from build123d import *

# Parameters (mm, degrees)
F1_DEPTH = 2
F2_R     = 2
F3_R     = 3.175
F4_DEPTH = 2
F5_W     = 50
F5_H     = 15
F6_DEPTH = 2


with BuildPart() as f1:
    # F0 (on Top) → F1 (new body)
    with BuildSketch(Plane.XY):
        Polygon((-8, -15), (8, -15), (8, 0), (25, 0), (25, 15), (-25, 15), (-25, 0), (-8, 0), align=None)
    extrude(amount=F1_DEPTH)

    # F2
    f2_edges = [f1.edges().sort_by_distance(p)[0] for p in [
        (-8, 0, 1),
        (8, 0, 1),
    ]]
    fillet(f2_edges, radius=F2_R)

    # F3 (on face) → F4 (join)
    with BuildSketch(Plane.XY.offset(2)):
        with BuildLine():
            ThreePointArc((-13.825, 7.5), (-17, 10.675), (-20.175, 7.5))
            ThreePointArc((-20.175, 7.5), (-17, 4.325), (-13.825, 7.5))
        make_face()
        with Locations((17, 7.5)):
            Circle(F3_R)
    extrude(amount=F4_DEPTH)

    # F5 (on face) → F6 (join)
    with BuildSketch(Plane(origin=(0, 0, 0), x_dir=(1, 0, 0), z_dir=(0, 0, -1))):
        with BuildLine():
            Line((8, 2), (8, 15))
            Line((8, 15), (-8, 15))
            Line((-8, 15), (-8, 2))
            ThreePointArc((-8, 2), (-8.585786, 0.585786), (-10, 0))
            Line((-10, 0), (-25, 0))
            Line((-25, 0), (-25, -15))
            Line((-25, -15), (25, -15))
            Line((25, -15), (25, 0))
            Line((25, 0), (10, 0))
            ThreePointArc((10, 0), (8.585786, 0.585786), (8, 2))
        make_face()
        with Locations((0, -22.5)):
            Rectangle(F5_W, F5_H)
    extrude(amount=F6_DEPTH)


solid = f1.part
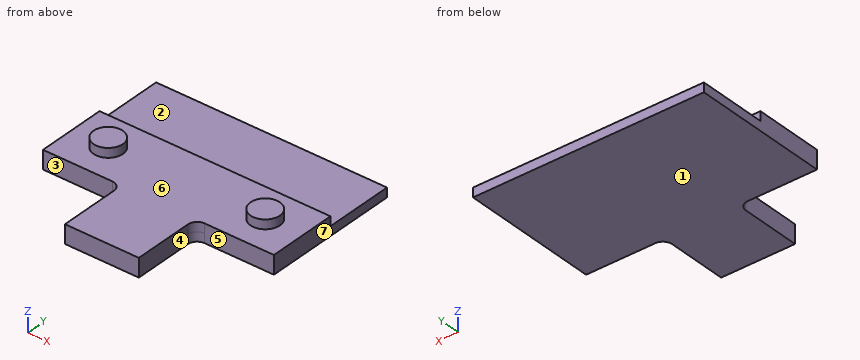
Could you check a few things on this model? Use its own coordinates, in mm. Face numbers are marked on the shaded views. A direction names the side the tool comes from. Give positions to 0.01 mm unless a question says otherwise; leave off trailing zeros. Write each loop counter-clockwise with the first axis right and the second up, starting at its lowest first coordinate (ties: lowest second). Pieces come first, ordered by that corner, then holes. Notation, with made-up numbers: (71.5, -12) -> (110.5, -12) arc R21 ccw to (110.5, 24) -> close; hole circle Ø2 at (-21.75, 77). An arc over 180 degrees is marked (long way). Write each question's results on one line, items separated by ' | '. Start each with the question number.
Q1. We'd pull the mould along X, two halves only. Please class the marked faces 5, 6 and 7: +X half, -X half, draft (parallel to the pull), parting line (faces both ways), or undercut.
Q2. Suppose I cut it at B-B, the plane z = 1.2. List the corners of the cut face in (x, y) for me, and give its area (3 significant figures).
Q3. Suppose I cut it at D-D, the plane x = 4. List the corners of the cut face in (y, z) for me.
Q4. I need wall thicknesses on probe 1 along Y at (x, z) = (-13.5, -0.15); probe 2 along Z at (x, y) = (11, 14); probe 3 along Z at (x, y) = (4, 20.5). Which ranges of each line are inside material? Lowest first, please.
Q5. I'm going to push flat-ended pins straight in: pin 1 Ø3 at (x, z) = (20.5, 0.5) entering from -Y; pin 2 Ø4.5 at (x, y) = (-4, 25.5) entering from +Z; pin 3 Ø2 at (y, z) = (-10, -0.5) entering from +X; pin 4 Ø24 at (x, y) = (-5, 3.5) entering from +Z. Where does each tip first touch, or does it pass through?
Q6. Which directions (+Z, -Z, +X, -X, +Y, -Y) give clear straight access to the entire face, cutting with the end or side of a thin tool? Please do the marked faces 1, 2, 3 and 4.
Q7. Suppose I cut it at C-C, the plane x = -17. List the corners of the cut face in (y, z) for me (3 decimals).
Q8. Suppose I cut it at A-A, the plane y = 7.5. List the corners of the cut face in (x, z) for me (3 decimals).
Outcome:
1) face 5: draft | face 6: undercut | face 7: +X half
2) outline: (-25, 0) -> (-10, 0) arc R2 cw to (-8, -2) -> (-8, -15) -> (8, -15) -> (8, -2) arc R2 cw to (10, 0) -> (25, 0) -> (25, 15) -> (-25, 15) -> close | area: 992 mm2
3) outline: (-15, -2) -> (30, -2) -> (30, 0) -> (15, 0) -> (15, 2) -> (-15, 2) -> close
4) probe 1: 0 to 30 | probe 2: -2 to 2 | probe 3: -2 to 0
5) pin 1: y = 0 | pin 2: z = 0 | pin 3: x = 8 | pin 4: z = 4
6) face 1: -Z, +X, -X, +Y, -Y | face 2: +Z, +X, -X, +Y | face 3: +Z, -Z, -X, -Y | face 4: +Z, -Z, +X, -Y
7) outline: (0, -2) -> (30, -2) -> (30, 0) -> (15, 0) -> (15, 2) -> (10.675, 2) -> (10.675, 4) -> (4.325, 4) -> (4.325, 2) -> (0, 2) -> close
8) outline: (-25, -2) -> (25, -2) -> (25, 2) -> (20.175, 2) -> (20.175, 4) -> (13.825, 4) -> (13.825, 2) -> (-13.825, 2) -> (-13.825, 4) -> (-20.175, 4) -> (-20.175, 2) -> (-25, 2) -> close
